Autodesk Inventor part; units mm, degrees
ref_plane "YZ Plane" through (0, 0, 0) normal (1, 0, 0) x (0, 1, 0)
ref_plane "XZ Plane" through (0, 0, 0) normal (0, 1, 0) x (-1, 0, 0)
ref_plane "XY Plane" through (0, 0, 0) normal (0, 0, 1) x (1, 0, 0)
sketch "Эскиз1" plane through (0, 0, 0) normal (0, 0, 1) x (1, 0, 0)
  line L0 (0, 3.5) -> (0, -3.5)
  line L1 (0, -3.5) -> (23, -3.5) construction
  line L2 (23, -3.5) -> (22.5, -3.2113)
  line L3 (22.5, -3.2113) -> (22.5, 2.5)
  line L4 (23.5, 3.5) -> (32, 3.5)
  line L5 (32, 3.5) -> (32, 0.6968)
  line L6 (32, 0.6968) -> (23, -3.5)
  line L7 (22.5, 2.5) -> (23.5, 3.5)
  point P0 (0, 0)
  point P1 (0, 0)
  point P2 (22.5, 3.5)
  dimension "d0" = 7
  dimension "d1" = 46
  dimension "d2" = 45
  dimension "d3" = 25
  dimension "d5" = 64
  dimension "d6" = 1
  dimension "d7" = 45
  dimension "d8" = 60
revolve "Вращение1" add sketch "Эскиз1" angle 360 about axis through (0, 3.5, 0) along (0, -1, 0)
sketch "Эскиз2" plane through (0, 3.5, 0) normal (0, 1, 0) x (1, 0, 0)
  line L0 (-3, 32) -> (3, 32)
  line L1 (3, 32) -> (3, 29)
  line L2 (3, 29) -> (-3, 29)
  line L3 (-3, 29) -> (-3, 32)
  circle A0 centre (0, 0) radius 32
  point P0 (0, 0)
  point P1 (0, 29)
  point P2 (3, 31.8591)
  point P3 (-3, 31.8591)
  dimension "d10" = 6
  dimension "d11" = 3
extrude "Выдавливание1" cut sketch "Эскиз2" against normal through all contours A0 L1 L2 L3 picked at (0, 30)
pattern_circular "Круговой массив1" count 4 over 360 about axis through (0, -0.3557, 0) along (0, -1, 0) of "Выдавливание1"
thread "Резьба1"
properties part number "76. Гайка первичного вала"
The model under review builds one solid part; all positions refer to its coordinate system, in mm. A direction names the side the tool comes from. Give positions to 0.01 mm unless a question says otherwise; leave off trailing zeros. Write each loop counter-clockwise with the first axis right and the second up, starting at its lowest first coordinate (ties: lowest second). Pieces come first, ordered by that corner, then holes. Notation, with made-up numbers: M 58.5,-11 L 96.5,-11 A12 cw 96.5,1 Z; hole C 23,-2.5 d7. An arc over 180 degrees is marked long. Answer in a Markdown table with one row per item.
Item 1: Tool access review of faces 1 (the face through (0, 1, 29)), 2 (the face through (-30, 2, -3)), 3 (the face through (30, 2, -3)): name each direction out of +Z, -Z, +X, -X, +Y, -Y from which nothing blocks a thin tool from reaching the whole face with its end or side.
Check sheet entries:
| item | result |
|---|---|
| face 1 | +Z, +Y, -Y |
| face 2 | -X, +Y, -Y |
| face 3 | +X, +Y, -Y |
Item 2: Add section A-A on z = 0. Give the boundary of the cut face in (x, y), plus the area to 3 significant figures.
Check sheet entries:
| item | result |
|---|---|
| outline | M -29,-0.7 L -23,-3.5 L -22.5,-3.21 L -22.5,2.5 L -23.5,3.5 L -29,3.5 Z; M 22.5,-3.21 L 23,-3.5 L 29,-0.7 L 29,3.5 L 23.5,3.5 L 22.5,2.5 Z |
| area | 73.1 mm2 |
Item 3: Add section B-B on x = 0. Give the boundary of the cut face in (y, z), plus the area to 3 significant figures.
Check sheet entries:
| item | result |
|---|---|
| outline | M -3.5,-23 L -0.7,-29 L 3.5,-29 L 3.5,-23.5 L 2.5,-22.5 L -3.21,-22.5 Z; M -3.5,23 L -3.21,22.5 L 2.5,22.5 L 3.5,23.5 L 3.5,29 L -0.7,29 Z |
| area | 73.1 mm2 |
Item 4: Draft analysis for pull direction X (two halves, no side actions). For faces 4 (the face through (10.382, -0.316, 19.961)), 5 (the face through (-30, 2, 3)), 6 (the face through (22.47, -3.24, -7.08)), 7 (the face through (-22.845, 2.079, -22.407)), state which applies: +X half, -X half, draft (parallel to the pull), parting line (faces both ways), or undercut.
Check sheet entries:
| item | result |
|---|---|
| face 4 | undercut |
| face 5 | draft |
| face 6 | parting line |
| face 7 | -X half |
Item 5: For line 1 along Z through (x, y) = (0, -0.55); line 2 along Z through (x, y) = (-14.5, 0); line 3 along Y through (x, z) = (-24, 8), list the stretches that pass through material, from the lowest coordinate up.
Check sheet entries:
| item | result |
|---|---|
| line 1 | -29 to -22.5, 22.5 to 29 |
| line 2 | -26.84 to -17.2, 17.2 to 26.84 |
| line 3 | -2.43 to 3.5 |
Item 6: Add section C-C on y = 1.5. Give the boundary of the cut face in (x, z).
Check sheet entries:
| item | result |
|---|---|
| outline | M -31.86,-3 A32 ccw -3,-31.86 L -3,-29 L 3,-29 L 3,-31.86 A32 ccw 31.86,-3 L 29,-3 L 29,3 L 31.86,3 A32 ccw 3,31.86 L 3,29 L -3,29 L -3,31.86 A32 ccw -31.86,3 L -29,3 L -29,-3 Z; hole C 0,0 d45 |
Item 7: For P1, Ø12, axis at x = 17, z = -10.5, coming from the -Y side; P2, Ø2.5, axis at y = 0.5, z = -30.5, coming from the -X side; P3, Ø2, axis at x = -1, y = 2.5, coming from the -Z side; P4, Ø3, axis at x = -30.5, y = 2, coming from the -Z side, all flat-tipped, find the tip position at first contact; note any pin that passes through.
Check sheet entries:
| item | result |
|---|---|
| P1 | y = -3.5 |
| P2 | x = -12.94 |
| P3 | z = -29 |
| P4 | z = -13.53 |
